The listing builds one solid part. Answer for the finished solid, in the listing's coordinates (mm). Face numbers are marked on the shaded views. Coordinates: 2 decimals unless noted, no trailing zeros. Write each loop counter-clockwise with the first axis right and the second up, starting at its lowest first coordinate (ties: lowest second). Pieces come first, ordered by that corner, then holes.
from build123d import *

# Parameters (mm, degrees)
SKETCH_2_W          = 807
SKETCH_2_H          = 307
EXTRUDE_1_DEPTH     = 25
SKETCH_3_W          = 801
SKETCH_3_H          = 301
CUT_EXTRUDE_1_DEPTH = 22
SKETCH_4_R          = 4
CUT_EXTRUDE_2_DEPTH = 308


with BuildPart() as part:
    # 草圖2 → 填料-伸長1 (new body)
    with BuildSketch(Plane(origin=(0, 0, 0), x_dir=(1, 0, 0), z_dir=(0, 1, 0))):
        with Locations((403.5, -153.5)):
            Rectangle(SKETCH_2_W, SKETCH_2_H)
    extrude(amount=EXTRUDE_1_DEPTH)

    # 草圖3 → 除料-伸長1 (cut)
    with BuildSketch(Plane(origin=(0, 25, 0), x_dir=(1, 0, 0), z_dir=(0, 1, 0))):
        with Locations((403.5, -153.5)):
            Rectangle(SKETCH_3_W, SKETCH_3_H)
    extrude(amount=-CUT_EXTRUDE_1_DEPTH, mode=Mode.SUBTRACT)

    # 草圖4 → 除料-伸長2 (cut, through all)
    with BuildSketch(Plane.XY.offset(307)):
        with Locations((759, 12.5)):
            Circle(SKETCH_4_R)
        with Locations((48, 12.5)):
            Circle(SKETCH_4_R)
    extrude(amount=-CUT_EXTRUDE_2_DEPTH, mode=Mode.SUBTRACT)


solid = part.part
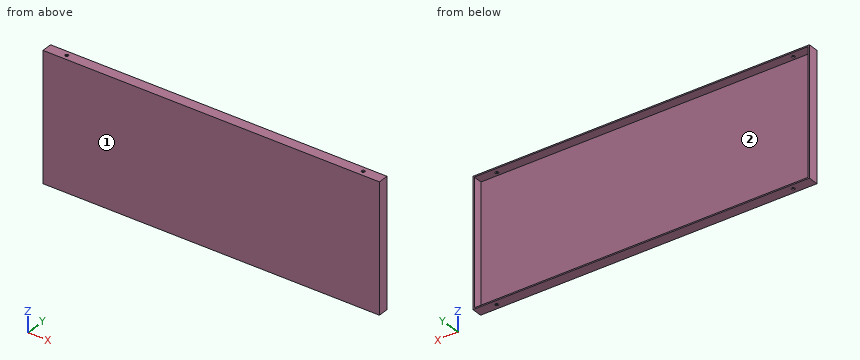
Q1. The part is cut by section B-B, the plane z = 24. Write down the section's boundary in (x, y).
Answers below:
outline: (0, 0) - (807, 0) - (807, 25) - (804, 25) - (804, 3) - (3, 3) - (3, 25) - (0, 25) - close
Q2. Given pin 1 (1 mm diameter, centred on x = 293.5, z = 213.5, fed in from +Y); pin 2 (5 mm diameter, centred on x = 759, y = 12.5, fed in from -Z), each flat-ended and moving along its own axis, determine where each tip first touches the part or whether it passes through.
Answers below:
pin 1: stops at y = 3
pin 2: passes through
Q3. Determine the mould class of the marked faces 1 and 2 for opening direction X: released by +X, released by -X, zero draft, split by the parting line, or undercut.
Answers below:
face 1: zero draft
face 2: undercut
Q4. Find the intervals of material crossed by probe 1 along Z at (x, y) = (64, 7.75); probe 2 along Y at (x, z) = (759, 1.1); probe 3 along X at (y, z) = (12, 139), in increasing order.
Answers below:
probe 1: z = 0 to 3, 304 to 307
probe 2: y = 0 to 8.5, 16.5 to 25
probe 3: x = 0 to 3, 804 to 807
Q5. The part is cut by section A-A, the plane y = 12.5. Write down the section's boundary in (x, z).
Answers below:
outline: (0, 0) - (44, 0) - (44, 3) - (3, 3) - (3, 304) - (44, 304) - (44, 307) - (0, 307) - close; (52, 0) - (755, 0) - (755, 3) - (52, 3) - close; (52, 304) - (755, 304) - (755, 307) - (52, 307) - close; (763, 0) - (807, 0) - (807, 307) - (763, 307) - (763, 304) - (804, 304) - (804, 3) - (763, 3) - close
Q6. The part is cut by section C-C, the plane x = 659.5. Write down the section's boundary in (y, z).
Answers below:
outline: (0, 0) - (25, 0) - (25, 3) - (3, 3) - (3, 304) - (25, 304) - (25, 307) - (0, 307) - close
